```python
from build123d import *

# Parameters (mm, degrees)
ESQUISSE2_R        = 1.05
BOSS_EXTRU_1_DEPTH = 100
ESQUISSE3_R        = 2.5
BOSS_EXTRU_2_DEPTH = 8
ESQUISSE4_R        = 5
BOSS_EXTRU_3_DEPTH = 42
CONG_4_R           = 1
CONG_5_R           = 1
CONG_6_R           = 1


with BuildPart() as part:
    # Esquisse2 → Boss.-Extru.1 (new body)
    with BuildSketch(Plane(origin=(0, 0, 0), x_dir=(1, 0, 0), z_dir=(0, 1, 0))):
        Circle(ESQUISSE2_R)
    extrude(amount=BOSS_EXTRU_1_DEPTH)

    # Esquisse3 → Boss.-Extru.2 (add)
    with BuildSketch(Plane(origin=(0, 100, 0), x_dir=(1, 0, 0), z_dir=(0, 1, 0))):
        Circle(ESQUISSE3_R)
    extrude(amount=-BOSS_EXTRU_2_DEPTH)

    # Esquisse4 → Boss.-Extru.3 (add)
    with BuildSketch(Plane.XZ.offset(-92)):
        Circle(ESQUISSE4_R)
    extrude(amount=BOSS_EXTRU_3_DEPTH)

    # Congé4
    cong_4_edges = [part.edges().sort_by_distance(p)[0] for p in [
        (-2.5, 100, 0),
    ]]
    fillet(cong_4_edges, radius=CONG_4_R)

    # Congé5
    cong_5_edges = [part.edges().sort_by_distance(p)[0] for p in [
        (-5, 92, 0),
    ]]
    fillet(cong_5_edges, radius=CONG_5_R)

    # Congé6
    cong_6_edges = [part.edges().sort_by_distance(p)[0] for p in [
        (-2.5, 92, 0),
    ]]
    fillet(cong_6_edges, radius=CONG_6_R)


solid = part.part
```
Can you work these out from the model? Positions are in its coordinate system, mm. A direction names the side the tool comes from. Give positions to 0.01 mm unless a question says otherwise; leave off trailing zeros. Write each loop counter-clockwise with the first axis right and the second up, starting at its lowest first coordinate (ties: lowest second). Pieces come first, ordered by that corner, then holes. Notation, with made-up numbers: (20, -29.5) -> (51, -29.5) arc R22 cw to (51, -15.5) -> close; hole circle Ø7 at (-15.75, 27.25). An arc over 180 degrees is marked (long way). Write item = value, one per line.
(1) Suppose I cut it at C-C on y = 49. Write out the boundary of the cut face in (x, z), then the cut area to 3 significant figures.
Worked out:
outline = circle Ø2.1 at (0, 0)
area = 3.46 mm^2
(2) I need wall thicknesses on probe 1 along Y at (x, z) = (-3.5, 1.25); probe 2 along Y at (x, z) = (1.25, 1); probe 3 along X at (y, z) = (76.5, -0.75). Which ranges of each line are inside material? Lowest first, please. Write a range as from..to.
Worked out:
probe_1 = 50..92
probe_2 = 50..99.99
probe_3 = -4.94..4.94
(3) Thinking about a two-plate mould opening in Y: for faces 3 (the face through (-0.1, 50, 1.2)), 4 (the face through (-0.54, 96.04, 2.44)), 5 (the face through (0, 100, 0)), which applies, released by +Y, released by -Y, zero draft, split by the parting line, or undercut?
Worked out:
face_3 = released by -Y
face_4 = zero draft
face_5 = released by +Y
(4) Suppose I cut it at A-A on z = 0. Write out the boundary of the cut face in (x, y), then the cut area to 3 significant figures.
Worked out:
outline = (-5, 50) -> (-1.05, 50) -> (-1.05, 0) -> (1.05, 0) -> (1.05, 50) -> (5, 50) -> (5, 91) arc R1 ccw to (4, 92) -> (3.5, 92) arc R1 cw to (2.5, 93) -> (2.5, 99) arc R1 ccw to (1.5, 100) -> (-1.5, 100) arc R1 ccw to (-2.5, 99) -> (-2.5, 93) arc R1 cw to (-3.5, 92) -> (-4, 92) arc R1 ccw to (-5, 91) -> close
area = 565 mm^2
(5) I'm going to push flat-ended pins straight in: P1, Ø1, axis at x = -2, z = -4, coming from the +Y side; P2, Ø1.5, axis at y = 25.5, z = -1, coming from the -X side; P3, Ø3, axis at x = -1, y = 14.5, coming from the +Z side. Where does each tip first touch, or does it pass through?
Worked out:
P1 = 92
P2 = -1.02
P3 = 1.05
(6) For faces 1 (the face through (-1.08, 70.79, -4.88)), 2 (the face through (1, 24.65, -0.32)), which set-ups out of +Z, -Z, +X, -X, +Y, -Y let a thin tool reach every point of the face, with its end or its side?
Worked out:
face_1 = +Y, -Y
face_2 = -Y
(7) Suppose I cut it at B-B on x = 0. Write out the boundary of the cut face in (y, z).
Worked out:
outline = (0, -1.05) -> (50, -1.05) -> (50, -5) -> (91, -5) arc R1 ccw to (92, -4) -> (92, -3.5) arc R1 cw to (93, -2.5) -> (99, -2.5) arc R1 ccw to (100, -1.5) -> (100, 1.5) arc R1 ccw to (99, 2.5) -> (93, 2.5) arc R1 cw to (92, 3.5) -> (92, 4) arc R1 ccw to (91, 5) -> (50, 5) -> (50, 1.05) -> (0, 1.05) -> close
